from build123d import *

# Parameters (mm, degrees)
SKETCH1_W               = 35.519995
SKETCH1_H               = 32.6499982
BOSS_EXTRUDE1_DEPTH     = 12.1700036
CUT_EXTRUDE1_DEPTH      = 29.893301397
CUT_EXTRUDE1_DEPTH_BACK = 5.2499768
SKETCH3_W               = 5.999988
SKETCH3_H               = 12.0000014
CUT_EXTRUDE2_DEPTH      = 2.999994
SKETCH4_W               = 23.5199936
SKETCH4_H               = 23.9599978
CUT_EXTRUDE3_DEPTH      = 6.4250062
CUT_EXTRUDE5_DEPTH      = 5.890006
CUT_EXTRUDE6_DEPTH      = 2.2999954
SKETCH8_R               = 1.7499965
CUT_EXTRUDE7_DEPTH      = 2.7999944


with BuildPart() as part:
    # Sketch1 → Boss-Extrude1 (new body)
    with BuildSketch(Plane(origin=(0, 0, 0), x_dir=(1, 0, 0), z_dir=(0, 1, 0))):
        with Locations((1.4404975, 1.509093805)):
            Rectangle(SKETCH1_W, SKETCH1_H)
    extrude(amount=BOSS_EXTRUDE1_DEPTH)

    # Sketch2 → Cut-Extrude1 (cut, two sides: drawn at the far end of the back side and taken through both)
    with BuildSketch(Plane(origin=(0, 12.1700036, 0), x_dir=(1, 0, 0), z_dir=(0, 1, 0)).offset(-CUT_EXTRUDE1_DEPTH_BACK)):
        Polygon((-13.8303, -9.315916295), (-15.995359179, -10.565913795), (-15.995359179, -13.065908795), (-13.8303, -14.315906295), (-11.665240821, -13.065908795), (-11.665240821, -10.565913795), align=None)
        Polygon((-11.665240821, 10.565913795), (-13.8303, 9.315916295), (-15.995359179, 10.565913795), (-15.995359179, 13.065908795), (-13.8303, 14.315906295), (-11.665240821, 13.065908795), align=None)
        Polygon((16.7005, 5.334067105), (14.535440821, 4.084069605), (14.535440821, 1.584074605), (16.7005, 0.334077105), (18.865559179, 1.584074605), (18.865559179, 4.084069605), align=None)
        Polygon((16.7005, -14.315906295), (18.865559179, -13.065908795), (18.865559179, -10.565913795), (16.7005, -9.315916295), (14.535440821, -10.565913795), (14.535440821, -13.065908795), align=None)
    extrude(amount=CUT_EXTRUDE1_DEPTH + CUT_EXTRUDE1_DEPTH_BACK, mode=Mode.SUBTRACT)

    # Sketch3 → Cut-Extrude2 (cut)
    with BuildSketch(Plane(origin=(0, 12.1700036, 0), x_dir=(1, 0, 0), z_dir=(0, 1, 0))):
        with Locations((16.200501, 11.834092205)):
            Rectangle(SKETCH3_W, SKETCH3_H)
    extrude(amount=-CUT_EXTRUDE2_DEPTH, mode=Mode.SUBTRACT)

    # Sketch4 → Cut-Extrude3 (cut)
    with BuildSketch(Plane(origin=(0, 12.1700036, 0), x_dir=(1, 0, 0), z_dir=(0, 1, 0))):
        with Locations((1.4404848, 3.054099605)):
            Rectangle(SKETCH4_W, SKETCH4_H)
    extrude(amount=-CUT_EXTRUDE3_DEPTH, mode=Mode.SUBTRACT)

    # Sketch6 → Cut-Extrude5 (cut)
    with BuildSketch(Plane.XY.offset(14.815905295)):
        with BuildLine():
            ThreePointArc((0.90468468, 8.436788325), (13.6504934, 12.1700036), (0.90468468, 15.903218875))
            ThreePointArc((0.90468468, 15.903218875), (-3.199511, 12.1700036), (0.90468468, 8.436788325))
        make_face()
    extrude(amount=-CUT_EXTRUDE5_DEPTH, mode=Mode.SUBTRACT)

    # Sketch7 → Cut-Extrude6 (cut)
    with BuildSketch(Plane.XY.offset(-15.034098505)):
        Polygon((8.9404952, 8.763635), (11.890496942, 10.4668193), (11.890496942, 13.8731879), (8.9404952, 15.5763722), (5.990493458, 13.8731879), (5.990493458, 10.4668193), align=None)
        Polygon((-6.0595002, 8.763635), (-3.109498458, 10.4668193), (-3.109498458, 13.8731879), (-6.0595002, 15.5763722), (-9.009501942, 13.8731879), (-9.009501942, 10.4668193), align=None)
    extrude(amount=-CUT_EXTRUDE6_DEPTH, mode=Mode.SUBTRACT)

    # Sketch8 → Cut-Extrude7 (cut)
    with BuildSketch(Plane(origin=(0, 0, -17.834092905), x_dir=(-1, 0, 0), z_dir=(0, 0, -1))):
        with Locations((-8.9404952, 12.1700036)):
            Circle(SKETCH8_R)
        with Locations((6.0595002, 12.1700036)):
            Circle(SKETCH8_R)
    extrude(amount=-CUT_EXTRUDE7_DEPTH, mode=Mode.SUBTRACT)


solid = part.part
Check sheet for the modelled part. Datum: model origin and axes. Units: mm. A direction names the side the tool comes from. Round coordinates to 2 decimals unless told otherwise and drop trailing zeros. Order: outer loops, then holes, each group sorted by start corner. A loop starts at its lowest first (then second) coordinate and runs counter-clockwise, first axis right, second up.
(1) Draft check along X on faces 3 (the cylindrical face through (-6.02, 10.42, -17.59)), 4 (the flat face through (16, 9.17, -12)), 5 (the flat face through (-11.665, 10, -12)). Enter one of: pulls with the +X half, pulls with the -X half, needs draft (parallel to the pull), parting line crosses it, or undercut.
(2) Cross-section at B-B, the plane x = 16. Enter the section's corners in (y, z).
(3) Go/stop test with flat-tipped pins: P1, Ø6.5, axis at x = 17, z = -12, coming from the +Y side; P2, Ø0.5, axis at y = 11.5, z = -16.5, coming from the +X side; P3, Ø1.3, axis at x = -14.5, z = 11, coming from the +Y side. Record where each tip stops, or that it passes through.
(4) Scan lines: probe 1 along X at (y, z) = (7.75, -13); probe 2 along X at (y, z) = (6.75, 8); probe 3 along Z at (x, y) = (-6, 8.5). Record each from-to range of solid material in increasing order.
(5) Cross-section at C-C, the plane x = -7. Enter the section's corners in (y, z) (3 decimals).
(6) Access from +Z, -Z, +X, -X, +Y, -Y to the whole of each face (thin tool, end or side, straight path). Record for faces 1 (the flat face through (15.6, 9.51, -0.97)), 2 (the flat face through (7.44, 9.63, -16.17)).
Check sheet entries:
1. face 3: undercut
1. face 4: needs draft
1. face 5: undercut
2. outline: (0, -17.83) - (9.17, -17.83) - (9.17, -5.83) - (12.17, -5.83) - (12.17, -4.93) - (6.92, -4.93) - (6.92, -0.74) - (12.17, -0.74) - (12.17, 9.72) - (6.92, 9.72) - (6.92, 13.91) - (12.17, 13.91) - (12.17, 14.82) - (0, 14.82) - close
3. P1: stops at y = 9.17
3. P2: stops at x = 13.2
3. P3: stops at y = 6.92
4. probe 1: x = -16.32 to -16, -11.67 to -10.32, 13.2 to 19.2
4. probe 2: x = -16.32 to -10.32, 13.2 to 19.2
4. probe 3: z = -17.83 to -15.03, 8.93 to 14.82
5. outline: (0, -17.834) - (10.694, -17.834) - (10.694, -17.334) - (9.307, -17.334) - (9.307, -15.034) - (5.745, -15.034) - (5.745, 8.926) - (12.17, 8.926) - (12.17, 14.816) - (0, 14.816) - close
6. face 1: +Y
6. face 2: +Z, +Y
